Autodesk Inventor part; units mm, degrees
ref_plane "YZ Plane" through (0, 0, 0) normal (1, 0, 0) x (0, 1, 0)
ref_plane "XZ Plane" through (0, 0, 0) normal (0, 1, 0) x (-1, 0, 0)
ref_plane "XY Plane" through (0, 0, 0) normal (0, 0, 1) x (1, 0, 0)
sketch "Sketch1" plane through (0, 0, 0) normal (0, 0, 1) x (1, 0, 0)
  line L0 (-14.5, -16) -> (14.5, -16)
  line L1 (14.5, -16) -> (14.5, 16)
  line L2 (14.5, 16) -> (-14.5, 16)
  line L3 (-14.5, 16) -> (-14.5, -16)
  line L4 (-14.5, -16) -> (14.5, 16) construction
  line L5 (14.5, -16) -> (-14.5, 16) construction
  line L6 (-6.5, -16) -> (-6.5, -7)
  line L7 (6.5, -7) -> (6.5, -16)
  line L8 (-6.5, -7) -> (6.5, -7)
  line L9 (-4.5, -1) -> (4.5, -1)
  line L10 (-4.5, 16) -> (-4.5, -1)
  line L11 (4.5, 16) -> (4.5, -1)
  point P0 (0, 0)
  dimension "d0" = 29
  dimension "d1" = 32
  dimension "d8" = 9
  dimension "d9" = 8
  dimension "d10" = 8
  dimension "d11" = 9
  dimension "d12" = 17
extrude "Extrusion1" add sketch "Sketch1" along normal blind 16 contours L3 L2 L10 L9 L11 L1 L0 L7 L8 L6
sketch "Sketch2" plane through (14.5, -16, 0) normal (1, 0, 0) x (0, 0, -1)
  line L0 (-16, 32) -> (-16, 0)
  line L1 (-16, 7) -> (0, 7)
  line L2 (0, 0) -> (-16, 0)
  line L3 (-16, 9) -> (-16, 0)
  line L4 (-16, 7) -> (-16, 0)
  line L5 (0, 0) -> (-16, 0)
  line L6 (-16, 0) -> (0, 0)
  line L7 (0, 0) -> (0, 7)
  line L8 (0, 0) -> (0, 9)
  point P0 (0, 16)
  dimension "d15" = 7
extrude "Extrusion2" add sketch "Sketch2" along normal blind 13
sketch "Sketch3" plane through (-14.5, -16, 0) normal (-1, 0, 0) x (0, 0, 1)
  line L0 (0, 0) -> (16, 0)
  line L1 (0, 0) -> (0, 7)
  line L2 (0, 0) -> (0, 7)
  line L3 (16, 7) -> (0, 7)
  line L4 (0, 7) -> (16, 7)
  line L5 (16, 7) -> (16, 0)
  line L6 (16, 0) -> (0, 0)
  point P0 (0, 16)
  dimension "d18" = 7
extrude "Extrusion3" add sketch "Sketch3" along normal blind 13
sketch "Sketch4" plane through (-14.5, 16, 0) normal (-1, 0, 0) x (0, 0, 1)
  circle A0 centre (8, -7) radius 3.5
  line L0 (0, 0) -> (16, 0)
  line L1 (16, 0) -> (16, -25)
  line L2 (0, 0) -> (0, -25)
  point P0 (0, -16)
  dimension "d21" = 7
  dimension "d22" = 7
  dimension "d23" = 16
  dimension "d24" = 8
extrude "Extrusion4" cut sketch "Sketch4" against normal through all
sketch "Sketch5" plane through (14.5, -9, 16) normal (0, 1, 0) x (1, 0, 0)
  line L0 (0, 0) -> (0, 16)
  line L1 (0, 0) -> (13, 0)
  line L2 (13, 16) -> (13, 0)
  line L3 (0, 16) -> (13, 16)
  line L4 (13, 16) -> (13, 6)
  line L5 (13, 0) -> (5.5, 0)
  line L6 (0, 0) -> (13, 0)
  line L7 (13, 16) -> (13, 0)
  line L8 (13, 0) -> (13, 6)
  circle A0 centre (6.5, 9.5) radius 3.5
  point P0 (-14.5, 16)
  dimension "d28" = 10
  dimension "d29" = 7.5
  dimension "d36" = 7
extrude "Extrusion5" cut sketch "Sketch5" against normal through all contours A0
sketch "Sketch6" plane through (14.5, -9, 16) normal (0, 1, 0) x (1, 0, 0)
  line L0 (-8, 0) -> (13, 0)
  line L1 (13, 0) -> (6.5, 0)
  line L2 (13, 0) -> (13, 7.5)
  line L3 (13, 0) -> (13, 16)
  line L4 (13, 7.5) -> (6.5, 0)
  point P0 (-14.5, 16)
  dimension "d39" = 6.5
  dimension "d40" = 7.5
extrude "Extrusion6" cut sketch "Sketch6" against normal through all
sketch "Sketch7" plane through (-14.5, -9, 16) normal (0, 1, 0) x (1, 0, 0)
  line L0 (8, 16) -> (-13, 16)
  line L1 (-13, 16) -> (-13, 0)
  circle A0 centre (-6.5, 9.5) radius 3.5
  line L2 (-13, 0) -> (-13, 7.5)
  line L3 (8, 0) -> (-13, 0)
  line L4 (-13, 0) -> (-6.5, 0)
  line L5 (-6.5, 0) -> (-13, 7.5)
  point P0 (14.5, 16)
  dimension "d44" = 7
  dimension "d46" = 7.5
  dimension "d47" = 6.5
extrude "Extrusion7" cut sketch "Sketch7" against normal through all contours A0
sketch "Sketch8" plane through (-14.5, -9, 16) normal (0, 1, 0) x (1, 0, 0)
  line L0 (8, 0) -> (-13, 0)
  line L1 (-13, 0) -> (-6.5, 0)
  line L2 (-6.5, 0) -> (-13, 0)
  line L3 (-13, 0) -> (-13, 7.5)
  line L4 (-13, 16) -> (-13, 0)
  line L5 (-13, 7.5) -> (-6.5, 0)
  point P0 (14.5, 16)
  dimension "d50" = 6.5
  dimension "d51" = 7.5
extrude "Extrusion8" cut sketch "Sketch8" against normal through all
properties part number "cad@26" material "Iron, Cast"
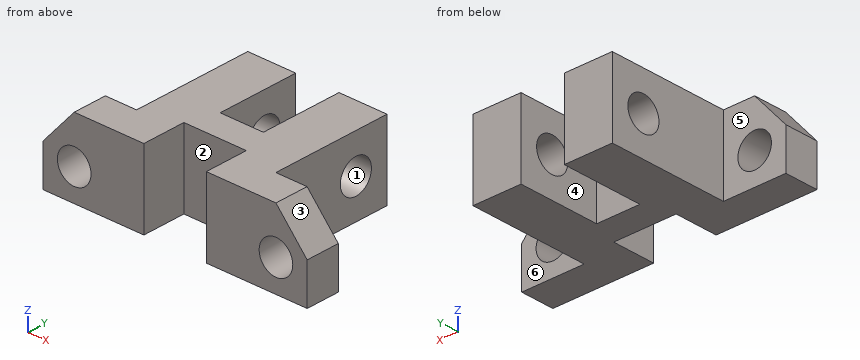
Design review of the part built by this model. Coordinates are the model's own, in mm. Face numbers are marked on the shaded views. A direction names the side the tool comes from. Round coordinates to 2 decimals unless told otherwise and drop trailing zeros. Write each loop counter-clockwise with the first axis right and the second up, starting at its lowest first coordinate (ties: lowest second). Pieces come first, ordered by that corner, then holes. Notation, with made-up numbers: (-25.5, 35.25) -> (0.5, 35.25) arc R22 ccw to (0.5, 64.25) -> close; hole circle Ø1 at (66, 34.25). An arc over 180 degrees is marked (long way). One line per item, written item: value. Start each with the question number.
Q1. Add section D-D (x = 7.5). Give the boundary of the cut face in (y, z).
Q2. Add section A-A (y = -11). Give the boundary of the cut face in (x, z), then the cut area to 3 significant figures.
Q3. The part is to be moulded in two halves that separate along X. For the marked faces 1, 2 and 3, say which applies: pulls with the +X half, pulls with the -X half, needs draft (parallel to the pull), parting line crosses it, or undercut.
Q4. Add section C-C (z = 14.5). Give the boundary of the cut face in (x, y), then the cut area to 3 significant figures.
Q5. To check wall thickness, follow probe 1 along X at (y, z) = (-12, 6.5); probe 2 along Z at (x, y) = (21, -10.25); probe 3 along Y at (x, z) = (10.5, 8). State the ranges of each line that lie inside material, in increasing order.
Q6. Add section B-B (y = 1.5). Give the boundary of the cut face in (x, z), then the cut area to 3 significant figures.
Q7. Tool access review of the marked faces 4, 5 and 6: name each direction out of +Z, -Z, +X, -X, +Y, -Y from which nothing blocks a thin tool from reaching the whole face with its end or side.
Q8. Insertion check: P1, Ø4.5, axis at y = -11, z = 10.5, coming from the +X side; P2, Ø4.5, axis at x = 0.5, z = 5.5, coming from the +Y side; P3, Ø9, axis at y = 9, z = 8, coming from the -X side; P4, Ø4, axis at x = 2, z = 10.5, coming from the -Y side. Each pin has a flat end and moves straight along its axis. Give the tip position at first contact, or say it passes through.
Response:
1. outline: (-16, 0) -> (16, 0) -> (16, 16) -> (-16, 16) -> close; hole circle Ø7 at (9, 8)
2. outline: (-27.5, 0) -> (-6.5, 0) -> (-6.5, 16) -> (-21, 16) -> (-27.5, 8.5) -> close; (6.5, 0) -> (27.5, 0) -> (27.5, 8.5) -> (21, 16) -> (6.5, 16) -> close; hole circle Ø7 at (-21, 6.5); hole circle Ø7 at (21, 6.5)
2. area: 546 mm^2
3. face 1: needs draft
3. face 2: undercut
3. face 3: pulls with the +X half
4. outline: (-22.3, -16) -> (-6.5, -16) -> (-6.5, -7) -> (6.5, -7) -> (6.5, -16) -> (22.3, -16) -> (22.3, -9) -> (14.5, -9) -> (14.5, 16) -> (4.5, 16) -> (4.5, -1) -> (-4.5, -1) -> (-4.5, 16) -> (-14.5, 16) -> (-14.5, -9) -> (-22.3, -9) -> close
4. area: 767 mm^2
5. probe 1: x = -27.5 to -24.5, -17.5 to -6.5, 6.5 to 17.5, 24.5 to 27.5
5. probe 2: z = 0 to 3, 10 to 16
5. probe 3: y = -16 to 5.5, 12.5 to 16
6. outline: (-14.5, 0) -> (-4.5, 0) -> (-4.5, 16) -> (-14.5, 16) -> close; (4.5, 0) -> (14.5, 0) -> (14.5, 16) -> (4.5, 16) -> close
6. area: 320 mm^2
7. face 4: +Z, -Z, +Y
7. face 5: +Z, -Z, -X, +Y
7. face 6: +Z, -Z, +X, +Y
8. P1: stops at x = 27.5
8. P2: stops at y = -1
8. P3: stops at x = -14.5
8. P4: stops at y = -7
